CAD build for the part. Positions are in the model's coordinates, mm. Coordinates: 2 decimals unless noted, no trailing zeros. Write each loop counter-clockwise with the first axis right and the second up, starting at its lowest first coordinate (ties: lowest second). Pieces come first, ordered by that corner, then holes. Notation, with made-up numbers: (1, 22.5) - (52, 22.5) arc R15 ccw to (52, 41.5) - close; hole circle Ø7 at (-37.5, -23). An arc over 180 degrees is marked (long way). Answer in a Markdown table with one row per item. Add a question column.
Q1. Band-saw the part on A-A (y = -124.5). List the corners of the cut face in (x, z).
Q2. Band-saw the part on B-B (z = -59). List the corners of the cut face in (x, y).
Q3. Pin check, flat tips, straight feed: pin 1 (1 mm diameter, centred on y = 393, z = -64, fed in from -X); pin 2 (1 mm diameter, centred on y = -71.5, z = -20.5, fed in from -X); pin 3 (6 mm diameter, centred on y = 280, z = -60, fed in from -X). Stop position of each tip, or through.
Q4. Drill centre lines: line 1 along X through (y, z) = (125, -6); line 2 along Z through (x, y) = (55.5, -57); line 3 along X through (y, z) = (25, -78.5). Where is each one in solid material? Low to high. Write a range as from..to.
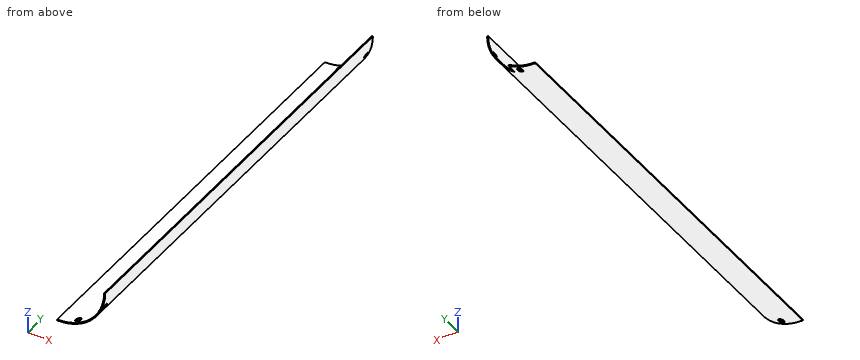
```python
from build123d import *

# Parameters (mm, degrees)
BOSS_EXTRUDE1_DEPTH     = 812
CUT_EXTRUDE2_REACH      = 820.409
CUT_EXTRUDE2_END_RADIUS = 90
SKETCH3_R               = 5.565
CUT_EXTRUDE3_REACH      = 820.409
CUT_EXTRUDE3_END_RADIUS = 90
SKETCH5_R               = 5.565
LPATTERN2_COUNT         = 2
LPATTERN2_PITCH         = 792
CUT_EXTRUDE5_DEPTH      = 20
BODY_MOVE_COPY1_ANGLE   = 180


with BuildPart() as part:
    # Sketch1 → Boss-Extrude1 (new body)
    with BuildSketch(Plane(origin=(0, 0, 0), x_dir=(1, 0, 0), z_dir=(0, 1, 0))):
        with BuildLine():
            Line((0, 92), (0, 90))
            ThreePointArc((0, 90), (63.639610307, 63.639610307), (90, 0))
            Line((90, 0), (92, 0))
            ThreePointArc((92, 0), (65.053823869, 65.053823869), (0, 92))
        make_face()
    extrude(amount=BOSS_EXTRUDE1_DEPTH)

    # Cut-Extrude2: up to this cylinder (the profile starts outside it)
    cut_extrude2_end = Plane(origin=(0, 10, 0), z_dir=(0, -1, 0)) * Cylinder(CUT_EXTRUDE2_END_RADIUS, 1821.818, mode=Mode.PRIVATE)
    # Sketch3 → Cut-Extrude2 (cut, up to the surface)
    with BuildSketch(Plane(origin=(84.996916991, 0, -35.206875778), x_dir=(-0.38268343236509045, 0, -0.9238795325112865), z_dir=(0.9238795325112865, 0, -0.38268343236509045)), mode=Mode.PRIVATE) as cut_extrude2_sk1:
        with Locations((0, 10)):
            Circle(SKETCH3_R)
    cut_extrude2_tool1 = extrude(cut_extrude2_sk1.sketch, amount=-CUT_EXTRUDE2_REACH, mode=Mode.PRIVATE) - cut_extrude2_end
    cut_extrude2 = cut_extrude2_tool1.solids().sort_by_distance((84.996917, 10, -35.206876))[0]
    add(cut_extrude2, mode=Mode.SUBTRACT)

    # Cut-Extrude3: up to this cylinder (the profile starts outside it)
    cut_extrude3_end = Plane(origin=(0, 10, 0), z_dir=(0, -1, 0)) * Cylinder(CUT_EXTRUDE3_END_RADIUS, 1821.818, mode=Mode.PRIVATE)
    # Sketch5 → Cut-Extrude3 (cut, up to the surface)
    with BuildSketch(Plane(origin=(35.206875778, 0, -84.996916991), x_dir=(-0.9238795325112878, 0, -0.3826834323650876), z_dir=(0.3826834323650876, 0, -0.9238795325112878)), mode=Mode.PRIVATE) as cut_extrude3_sk1:
        with Locations((0, 10)):
            Circle(SKETCH5_R)
    cut_extrude3_tool1 = extrude(cut_extrude3_sk1.sketch, amount=-CUT_EXTRUDE3_REACH, mode=Mode.PRIVATE) - cut_extrude3_end
    cut_extrude3 = cut_extrude3_tool1.solids().sort_by_distance((35.206876, 10, -84.996917))[0]
    add(cut_extrude3, mode=Mode.SUBTRACT)

    # LPattern2: Cut-Extrude2, Cut-Extrude3 ×2
    with Locations(*[(0, i * LPATTERN2_PITCH, 0) for i in range(1, LPATTERN2_COUNT)]):
        add(cut_extrude2, mode=Mode.SUBTRACT)
        add(cut_extrude3, mode=Mode.SUBTRACT)

    # Sketch7 → Cut-Extrude5 (cut)
    with BuildSketch(Plane.XZ):
        with BuildLine():
            Line((76.447375943, -51.183969281), (74.784435976, -50.072828318))
            ThreePointArc((74.784435976, -50.072828318), (63.639610307, -63.639610307), (50.072828318, -74.784435976))
            Line((50.072828318, -74.784435976), (51.183969281, -76.447375943))
            ThreePointArc((51.183969281, -76.447375943), (65.053823869, -65.053823869), (76.447375943, -51.183969281))
        make_face()
    extrude(amount=-CUT_EXTRUDE5_DEPTH, mode=Mode.SUBTRACT)


with BuildPart() as part_1:
    # Body-Move/Copy1: moved
    add(part.part.moved(Location((0, 0, 0))).rotate(Axis((0, 252, 0), (0.7071067811865488, -4.937700262164522e-15, -0.7071067811865462)), BODY_MOVE_COPY1_ANGLE))


solid = part_1.part
```
Checked values:
| question | item | result |
|---|---|---|
| 1 | outline | (0, -92) arc R92 ccw to (92, 0) - (90, 0) arc R90 cw to (0, -90) - close |
| 2 | outline | (67.96, -308) - (70.59, -308) - (70.59, 484) - (67.96, 484) - close |
| 3 | pin 1 | stops at x = 62.77 |
| 3 | pin 2 | stops at x = 87.52 |
| 3 | pin 3 | stops at x = 64.27 |
| 4 | line 1 | x = 89.8..91.8 |
| 4 | line 2 | z = -73.37..-70.85 |
| 4 | line 3 | x = 44.02..47.98 |
